Model file for the job. Use its own axes, mm. A direction names the side the tool comes from. Round coordinates to 2 decimals unless told otherwise and drop trailing zeros. Loops run counter-clockwise (first coordinate to the right, second up) from the corner with the lowest first, then second, coordinate; pieces in that order, holes last. Notation, with made-up numbers: M -9,-31 L 22,-31 A33 cw 22,7 Z; hole C 37.25,29 d7. An arc over 180 degrees is marked long. Answer in a Markdown table with one row per item.
from build123d import *

# Parameters (mm, degrees)
SALIENTE_EXTRUIR2_DEPTH      = 26.5
SALIENTE_EXTRUIR2_DEPTH_BACK = 1
CROQUIS1_R                   = 34
CROQUIS1_R_2                 = 24
CROQUIS2_R                   = 7
SALIENTE_EXTRUIR3_DEPTH      = 30
SALIENTE_EXTRUIR4_DEPTH      = 13


with BuildPart() as part:
    # Croquis1 → Saliente-Extruir2 (new, two sides: drawn at the far end of the back side and taken through both)
    with BuildSketch(Plane.XY.offset(-SALIENTE_EXTRUIR2_DEPTH_BACK)):
        Circle(CROQUIS1_R)
        Circle(CROQUIS1_R_2, mode=Mode.SUBTRACT)
    extrude(amount=SALIENTE_EXTRUIR2_DEPTH + SALIENTE_EXTRUIR2_DEPTH_BACK)



with BuildPart() as body_2:
    # Croquis2 → Saliente-Extruir3 (new body)
    with BuildSketch(Plane.XY):
        Circle(CROQUIS2_R)
    extrude(amount=SALIENTE_EXTRUIR3_DEPTH)


with BuildPart() as part_1:
    add(part.part)

    add(body_2.part)  # Saliente-Extruir4 merges body 2
    # Croquis3 → Saliente-Extruir4 (add)
    with BuildSketch(Plane.XY):
        with BuildLine():
            ThreePointArc((5.215852398, 23.426371545), (0, 24), (-5.215852398, 23.426371545))
            Line((-5.215852398, 23.426371545), (0, 0))
            Line((0, 0), (5.215852398, 23.426371545))
        make_face()
        with BuildLine():
            Line((-23.891590342, 2.278576513), (0, 0))
            Line((0, 0), (-20.66801628, 12.199717335))
            ThreePointArc((-20.66801628, 12.199717335), (-22.825356391, 7.416407865), (-23.891590342, 2.278576513))
        make_face()
        with BuildLine():
            Line((20.66801628, 12.199717335), (0, 0))
            Line((0, 0), (23.891590342, 2.278576513))
            ThreePointArc((23.891590342, 2.278576513), (22.825356391, 7.416407865), (20.66801628, 12.199717335))
        make_face()
        with BuildLine():
            Line((17.989388939, -15.886531579), (0, 0))
            Line((0, 0), (9.549962479, -22.018133814))
            ThreePointArc((9.549962479, -22.018133814), (14.106846055, -19.416407865), (17.989388939, -15.886531579))
        make_face()
        with BuildLine():
            Line((-9.549962479, -22.018133814), (0, 0))
            Line((0, 0), (-17.989388939, -15.886531579))
            ThreePointArc((-17.989388939, -15.886531579), (-14.106846055, -19.416407865), (-9.549962479, -22.018133814))
        make_face()
    extrude(amount=SALIENTE_EXTRUIR4_DEPTH)


solid = part_1.part
1. Tool access for faces 1 (the flat face through (7.1, 23.1, -1)), 2 (the flat face through (10, -13, 13)), 3 (the flat face through (0, 1, 0)), 4 (the flat face through (3.34, 15.01, 6.41)): list every direction of +Z, -Z, +X, -X, +Y, -Y with a clear straight run to the whole face (end or side of a thin tool).
Verdict:
| item | result |
|---|---|
| face 1 | -Z, +X, -X, +Y, -Y |
| face 2 | +Z |
| face 3 | -Z |
| face 4 | +Z, -Z |
2. Wall check: probe 1 along Y at (x, z) = (0, 19.5); probe 2 along Y at (x, z) = (-16.5, 6); probe 3 along Y at (x, z) = (0, 9). Give the ranges that are in metal, low to high.
Verdict:
| item | result |
|---|---|
| probe 1 | y = -34 to -24, -7 to 7, 24 to 34 |
| probe 2 | y = -29.73 to -14.57, 1.57 to 9.74, 17.43 to 29.73 |
| probe 3 | y = -34 to -24, -7 to 34 |
3. Mould opens along Y. For faces 5 (the flat face through (0, 0, 30)), 6 (the cylindrical face through (18.28, 28.67, 12.56)), 7 (the flat face through (15.31, 1.46, 6.41)) say: +Y half, -Y half, draft (parallel to the pull), parting line (faces both ways), or undercut.
Verdict:
| item | result |
|---|---|
| face 5 | draft |
| face 6 | parting line |
| face 7 | undercut |
4. Saw through at D-D (z = 19). Write the cut outline in (x, y), and give its area (3 significant figures).
Verdict:
| item | result |
|---|---|
| outline | C 0,0 d68; C 0,0 d14; hole C 0,0 d48 |
| area | 1,980 mm² |
5. Saw through at B-B (x = 0). Write the cut outline in (y, z), and give its area (3 significant figures).
Verdict:
| item | result |
|---|---|
| outline | M -34,-1 L -24,-1 L -24,26.5 L -34,26.5 Z; M -7,0 L 24,0 L 24,-1 L 34,-1 L 34,26.5 L 24,26.5 L 24,13 L 7,13 L 7,30 L -7,30 Z |
| area | 1,190 mm² |
6. Pin check, flat tips, straight feed: pin 1 (8 mm diameter, centred on x = -11, y = 2, fed in from +Z); pin 2 (1 mm diameter, centred on x = -2.5, z = 12, fed in from +Y); pin 3 (12 mm diameter, centred on x = -10.5, z = 22.5, fed in from +Y); pin 4 (20.5 mm diameter, centred on x = 13, y = 11, fed in from +Z). Stop position of each tip, or through.
Verdict:
| item | result |
|---|---|
| pin 1 | stops at z = 13 |
| pin 2 | stops at y = 33.94 |
| pin 3 | stops at y = 33.7 |
| pin 4 | stops at z = 30 |
7. Saw through at C-C (y = -2.5). Write the cut outline in (x, z), and give its area (3 significant figures).
Verdict:
| item | result |
|---|---|
| outline | M -33.91,-1 L -23.87,-1 L -23.87,26.5 L -33.91,26.5 Z; M -6.54,0 L 6.54,0 L 6.54,30 L -6.54,30 Z; M 23.87,-1 L 33.91,-1 L 33.91,26.5 L 23.87,26.5 Z |
| area | 944 mm² |
8. Saw through at A-A (y = -13.5). Write the cut outline in (x, z).
Verdict:
| item | result |
|---|---|
| outline | M -31.2,-1 L -19.84,-1 L -19.84,26.5 L -31.2,26.5 Z; M -15.29,0 L -5.86,0 L -5.86,13 L -15.29,13 Z; M 5.86,0 L 15.29,0 L 15.29,13 L 5.86,13 Z; M 19.84,-1 L 31.2,-1 L 31.2,26.5 L 19.84,26.5 Z |
